The listing builds one solid part. Answer for the finished solid, in the listing's coordinates (mm). Face numbers are marked on the shaded views. A direction names the side the tool comes from. Coordinates: 2 decimals unless noted, no trailing zeros. Order: outer loops, then holes, each group sorted by start corner. A loop starts at its lowest first (then second) coordinate and runs counter-clockwise, first axis right, second up. Notation, with made-up numbers: (70, -16) - (90, -16) arc R22 cw to (90, 13) - close; hole circle Ø1 at (76, -9.75). An arc over 180 degrees is marked (long way). Use a Markdown table: item, result. Add a question column.
Item 1: Flat-ended cylindrical pins translate along their axes: P1, Ø1.9, axis at x = 51, z = 21.5, coming from the -Y side; P2, Ø3.5, axis at y = 15.5, z = 6.22, coming from the +X side; P3, Ø11.5, axis at y = 8.5, z = 15, coming from the -X side. Find the tip coordinate at first contact, or state that the pin passes through.
Item 2: The part is cut by section C-C, the plane y = 15.5. State how many separate pieces and enclosed holes the cut face has, then the cut area to 3 significant figures.
Item 3: Find the intervals of material crossed by line 1 along Z through (x, y) = (52.3, -15.5); line 2 along X through (y, z) = (12, 26.5); line 3 along Z through (x, y) = (51, -15), in increasing order.
Item 4: The part is cut by section B-B, the plane x = 0. Give the vertices of the cut face in (y, z).
Item 5: For the marked faces 1, 2 and 3, determine the directions among +Z, -Z, +X, -X, +Y, -Y from which every point of the face is accessible in a straight line to the end or side of a thin tool.
Item 6: The part is cut by section A-A, the plane z = 24. Give the vertices of the cut face in (x, y).
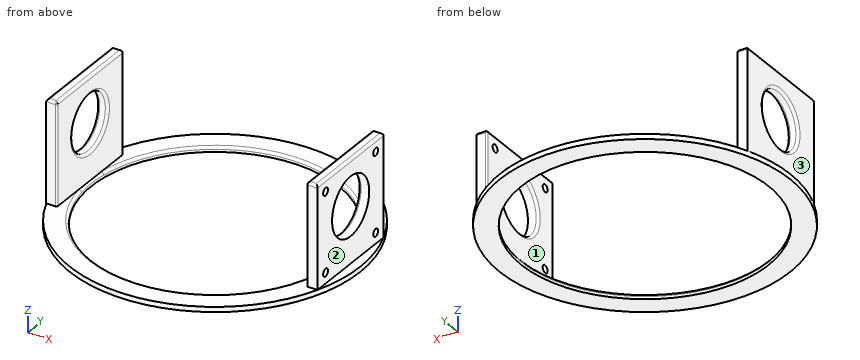
from build123d import *

# Parameters (mm, degrees)
SKETCH_R        = 57
SKETCH_R_2      = 48.5
PAD_DEPTH       = 2
SKETCH001_W     = 4.21681
SKETCH001_H     = 41
SKETCH001_W_2   = 4.21
PAD001_DEPTH    = 40
SKETCH002_R     = 1.5
SKETCH002_R_2   = 11.5
POCKET_DEPTH    = 5
SKETCH003_R     = 11
POCKET001_DEPTH = 5
FILLET_R        = 1
FILLET001_R     = 1
FILLET002_R     = 0.5
FILLET003_R     = 0.5
FILLET004_R     = 0.5
FILLET005_R     = 1
FILLET006_R     = 1
FILLET007_R     = 1
FILLET008_R     = 1


with BuildPart() as part:
    # Sketch → Pad (new body)
    with BuildSketch(Plane.XY):
        Circle(SKETCH_R)
        Circle(SKETCH_R_2, mode=Mode.SUBTRACT)
    extrude(amount=PAD_DEPTH)

    # Sketch001 → Pad001 (new body)
    with BuildSketch(Plane.XY.offset(2)):
        with Locations((-51.108405, 0)):
            Rectangle(SKETCH001_W, SKETCH001_H)
        with Locations((51.105, 0)):
            Rectangle(SKETCH001_W_2, SKETCH001_H)
    extrude(amount=PAD001_DEPTH)

    # Sketch002 → Pocket (cut)
    with BuildSketch(Plane.YZ.offset(53.21)):
        with Locations((-15.5, 6.218866)):
            Circle(SKETCH002_R)
        with Locations((-15.5, 37.218866)):
            Circle(SKETCH002_R)
        with Locations((15.5, 37.218866)):
            Circle(SKETCH002_R)
        with Locations((15.5, 6.218866)):
            Circle(SKETCH002_R)
        with Locations((0, 24)):
            Circle(SKETCH002_R_2)
    extrude(amount=-POCKET_DEPTH, mode=Mode.SUBTRACT)

    # Sketch003 → Pocket001 (cut)
    with BuildSketch(Plane(origin=(-53.21681, 0, 0), x_dir=(0, -1, 0), z_dir=(-1, 0, 0))):
        with Locations((0, 24)):
            Circle(SKETCH003_R)
    extrude(amount=-POCKET001_DEPTH, mode=Mode.SUBTRACT)

    # Fillet
    fillet_edges = [part.edges().sort_by_distance(p)[0] for p in [
        (51.105, 20.5, 42),
        (53.21, 0, 42),
        (51.105, -20.5, 42),
        (49, 0, 42),
    ]]
    fillet(fillet_edges, radius=FILLET_R)

    # Fillet001
    fillet001_edges = [part.edges().sort_by_distance(p)[0] for p in [
        (-51.108405, 20.5, 42),
        (-49, 0, 42),
        (-51.108405, -20.5, 42),
        (-53.21681, 0, 42),
    ]]
    fillet(fillet001_edges, radius=FILLET001_R)

    # Fillet002
    fillet002_edges = [part.edges().sort_by_distance(p)[0] for p in [
        (-49, 20.5, 21.5),
    ]]
    fillet(fillet002_edges, radius=FILLET002_R)

    # Fillet003
    fillet003_edges = [part.edges().sort_by_distance(p)[0] for p in [
        (49, 20.5, 21.5),
    ]]
    fillet(fillet003_edges, radius=FILLET003_R)

    # Fillet004
    fillet004_edges = [part.edges().sort_by_distance(p)[0] for p in [
        (-49, -20.5, 21.5),
        (49, -20.5, 21.5),
    ]]
    fillet(fillet004_edges, radius=FILLET004_R)

    # Fillet005
    fillet005_edges = [part.edges().sort_by_distance(p)[0] for p in [
        (-49, 11, 24),
    ]]
    fillet(fillet005_edges, radius=FILLET005_R)

    # Fillet006
    fillet006_edges = [part.edges().sort_by_distance(p)[0] for p in [
        (49, -11.5, 24),
    ]]
    fillet(fillet006_edges, radius=FILLET006_R)

    # Fillet007
    fillet007_edges = [part.edges().sort_by_distance(p)[0] for p in [
        (-53.21681, 11, 24),
    ]]
    fillet(fillet007_edges, radius=FILLET007_R)

    # Fillet008
    fillet008_edges = [part.edges().sort_by_distance(p)[0] for p in [
        (-48.5, 0, 2),
    ]]
    fillet(fillet008_edges, radius=FILLET008_R)


solid = part.part
Solution:
| question | item | result |
|---|---|---|
| 1 | P1 | stops at y = -20.5 |
| 1 | P2 | stops at x = 53.21 |
| 1 | P3 | stops at x = -53.22 |
| 2 | separate pieces | 4 |
| 2 | enclosed holes | 0 |
| 2 | area | 346 mm2 |
| 3 | line 1 | z = 0 to 4.72, 7.72 to 35.72, 38.72 to 42 |
| 3 | line 2 | x = -53.22 to -49, 49.03 to 53.21 |
| 3 | line 3 | z = 0 to 4.8, 7.63 to 35.8, 38.63 to 42 |
| 4 | outline | (-57, 0) - (-48.5, 0) - (-48.5, 1) arc R1 ccw to (-49.5, 2) - (-57, 2) - close; (48.5, 0) - (57, 0) - (57, 2) - (49.5, 2) arc R1 ccw to (48.5, 1) - close |
| 5 | face 1 | +Z, +Y, -Y |
| 5 | face 2 | +Z, +X, +Y, -Y |
| 5 | face 3 | +Z, -X, +Y, -Y |
| 6 | outline | (-53.22, -20.5) - (-49.5, -20.5) arc R0.5 ccw to (-49, -20) - (-49, -12) arc R1 ccw to (-50, -11) - (-52.22, -11) arc R1 ccw to (-53.22, -12) - close; (-53.22, 12) arc R1 ccw to (-52.22, 11) - (-50, 11) arc R1 ccw to (-49, 12) - (-49, 20) arc R0.5 ccw to (-49.5, 20.5) - (-53.22, 20.5) - close; (49, -20) arc R0.5 ccw to (49.5, -20.5) - (53.21, -20.5) - (53.21, -11.5) - (50, -11.5) arc R1 ccw to (49, -12.5) - close; (49, 12.5) arc R1 ccw to (50, 11.5) - (53.21, 11.5) - (53.21, 20.5) - (49.5, 20.5) arc R0.5 ccw to (49, 20) - close |
